Read the model definition and answer for the solid it produces. Units are mm, in the model's axes. Face numbers are marked on the shaded views. A direction names the side the tool comes from. Coordinates: 2 decimals unless noted, no trailing zeros. Write each loop counter-clockwise with the first axis right and the second up, starting at its lowest first coordinate (ties: lowest second). Pieces come first, ordered by that corner, then holes.
(1) Find the intervals of material crossed by probe 1 along Z at (x, y) = (60.5, 0.75); probe 2 along Y at (x, z) = (52, 4.5); probe 3 along Y at (x, z) = (75.5, 5.5), in increasing order.
(2) Given pin 1 (5.5 mm diameter, centred on x = 78, y = 13.5, fed in from -Z); pin 2 (4 mm diameter, centred on y = -4.5, z = 1.5, fed in from -X); pin 3 (3 mm diameter, centred on x = 46.63, y = 14.15, fed in from +Z), each flat-ended and moving along its own axis, determine where each tip first touches the part or whether it passes through.
(3) The mould has two halves that part along Y. Classify the marked faces 4, 5, 6 and 7: +Y half, -Y half, draft (parallel to the pull), parting line (faces both ways), or undercut.
(4) Section B-B on x = 61.5 is taken. Write down the section's boundary in (y, z).
(5) Section A-A on z = 2.25 is taken. Write down the section's boundary in (x, y).
(6) Section C-C on y = 10.25 is taken. Write down the section's boundary in (x, z), then the cut area to 3 significant figures.
(7) Section D-D on y = -8.25 is taken. State how many separate pieces and enclosed holes the cut face has, then the cut area to 3 significant figures.
(8) Which of the six approach directions +Z, -Z, +X, -X, +Y, -Y give full straight-line access (tool end or side, diameter ignored) to the marked faces 1, 2 and 3?
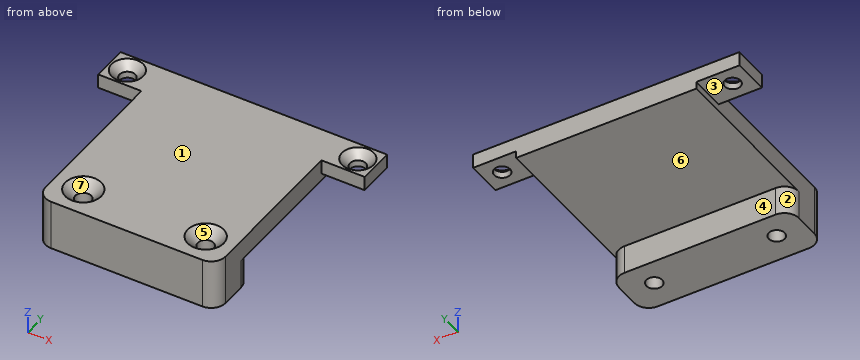
Autodesk Inventor part; units mm, degrees
ref_plane "YZ Plane" through (0, 0, 0) normal (1, 0, 0) x (0, 1, 0)
ref_plane "XZ Plane" through (0, 0, 0) normal (0, 1, 0) x (-1, 0, 0)
ref_plane "XY Plane" through (0, 0, 0) normal (0, 0, 1) x (1, 0, 0)
sketch "Skizze1" plane through (0, 0, 0) normal (0, 0, 1) x (1, 0, 0)
  line L0 (75.1333, -4.3546) -> (75.1333, -11.8546)
  line L1 (75.1333, -11.8546) -> (50.1333, -11.8546)
  line L2 (50.1333, -11.8546) -> (50.1333, -4.3546)
  line L3 (50.1333, -4.3546) -> (75.1333, -4.3546)
  point P0 (0, 0)
  dimension "d1" = 7.5
  dimension "d2" = 25
extrude "Extrusion1" add sketch "Skizze1" along normal blind 4
sketch "Skizze2" plane through (0, 0, 4) normal (0, 0, 1) x (1, 0, 0)
  line L0 (75.1333, 16.6454) -> (50.1333, 16.6454)
  line L1 (50.1333, 16.6454) -> (50.1333, -4.3546)
  line L2 (75.1333, -4.3546) -> (75.1333, 16.6454)
  line L3 (50.1333, -11.8546) -> (75.1333, -11.8546)
  line L4 (75.1333, -11.8546) -> (75.1333, -4.3546)
  line L5 (50.1333, -4.3546) -> (50.1333, -11.8546)
  line L6 (50.1333, 16.6454) -> (45.1333, 16.6454)
  line L7 (45.1333, 16.6454) -> (45.1333, 11.6454)
  line L8 (45.1333, 11.6454) -> (50.1333, 11.6454)
  line L9 (50.1333, 11.6454) -> (50.1333, 16.6454)
  line L10 (75.1333, 16.6454) -> (80.1333, 16.6454)
  line L11 (80.1333, 16.6454) -> (80.1333, 11.6454)
  line L12 (80.1333, 11.6454) -> (75.1333, 11.6454)
  line L13 (75.1333, 11.6454) -> (75.1333, 16.6454)
  point P0 (0, 0)
  dimension "d25" = 28.5
  dimension "d28" = 5
  dimension "d29" = 5
extrude "Extrusion2" add sketch "Skizze2" along normal blind 3 contours L2 L4 L3 L5 L1 L0
sketch "Skizze3" plane through (0, 0, 7) normal (0, 0, 1) x (1, 0, 0)
  line L0 (50.1333, 16.6454) -> (50.1333, -11.8546)
  line L1 (54.1333, -7.8546) -> (50.1333, -7.8546) construction
  line L2 (54.1333, -7.8546) -> (54.1333, -11.8546) construction
  line L3 (71.1333, -7.8546) -> (71.1333, -11.8546) construction
  line L4 (71.1333, -7.8546) -> (75.1333, -7.8546) construction
  line L5 (50.1333, -11.8546) -> (75.1333, -11.8546) construction
  line L6 (75.1333, -11.8546) -> (75.1333, 16.6454) construction
  point P0 (0, 0)
  dimension "d26" = 4
hole "Bohrung1" at (54.1333, -7.8546, 7) at (71.1333, -7.8546, 7) direction (0, 0, -1) diameter 2.2 end through all countersink diameter 5 countersink angle 90
fillet "Rundung1" radius 2 4 edges at (50.1333, -11.8546, 3.5) (75.1333, -11.8546, 3.5) (75.1333, -4.3546, 2) (50.1333, -4.3546, 2)
sketch "Skizze4" plane through (0, 0, 7) normal (0, 0, 1) x (1, 0, 0)
  line L0 (75.1333, -6.3546) -> (75.1333, 16.6454)
  line L1 (81.1333, 16.6454) -> (75.1333, 16.6454)
  line L2 (75.1333, 16.6454) -> (75.1333, 11.6454)
  line L3 (75.1333, 11.6454) -> (81.1333, 11.6454)
  line L4 (81.1333, 11.6454) -> (81.1333, 16.6454)
  line L5 (75.1333, 16.6454) -> (50.1333, 16.6454)
  line L6 (50.1333, 16.6454) -> (44.1333, 16.6454)
  line L7 (44.1333, 16.6454) -> (44.1333, 11.6454)
  line L8 (44.1333, 11.6454) -> (50.1333, 11.6454)
  line L9 (50.1333, 11.6454) -> (50.1333, 16.6454)
  point P0 (0, 0)
  dimension "d30" = 5
  dimension "d31" = 6
extrude "Extrusion3" add sketch "Skizze4" against normal blind 2
sketch "Skizze5" plane through (0, 0, 7) normal (0, 0, 1) x (1, 0, 0)
  line L0 (44.1333, 11.6454) -> (44.1333, 16.6454)
  line L1 (44.1333, 14.1454) -> (46.6333, 14.1454)
  line L2 (78.6333, 14.1454) -> (81.1333, 14.1454)
  line L3 (81.1333, 11.6454) -> (81.1333, 16.6454)
  line L4 (44.1333, 11.6454) -> (50.1333, 11.6454)
  point P0 (0, 0)
  dimension "d34" = 2.5
  dimension "d42" = 2.5
  dimension "d43" = 2.5
hole "Bohrung2" at (78.6333, 14.1454, 7) at (46.6333, 14.1454, 7) direction (0, 0, -1) diameter 2.2 end through all countersink diameter 4.4 countersink angle 90
properties part number "Sliderhalter" material "PC/ABS-Kunststoff, 3DDruck, PLA"
Response:
1. probe 1: z = 4 to 7
1. probe 2: y = -11.85 to 16.65
1. probe 3: y = 11.65 to 16.65
2. pin 1: stops at z = 5
2. pin 2: stops at x = 50.13
2. pin 3: stops at z = 6.31
3. face 4: +Y half
3. face 5: undercut
3. face 6: draft
3. face 7: undercut
4. outline: (-11.85, 0) - (-4.35, 0) - (-4.35, 4) - (16.65, 4) - (16.65, 7) - (-11.85, 7) - close
5. outline: (50.13, -9.85) arc R2 ccw to (52.13, -11.85) - (73.13, -11.85) arc R2 ccw to (75.13, -9.85) - (75.13, -6.35) arc R2 ccw to (73.13, -4.35) - (52.13, -4.35) arc R2 ccw to (50.13, -6.35) - close; hole circle Ø2.2 at (54.13, -7.85); hole circle Ø2.2 at (71.13, -7.85)
6. outline: (50.13, 4) - (75.13, 4) - (75.13, 7) - (50.13, 7) - close
6. area: 75.0 mm2
7. separate pieces: 3
7. enclosed holes: 0
7. area: 142 mm2
8. face 1: +Z, +X, -X, +Y, -Y
8. face 2: -Z, -X, +Y
8. face 3: -Z, -X, +Y, -Y
